Model file for the job. Use its own axes, mm. Face numbers are marked on the shaded views. A direction names the side the tool comes from. Give positions to 0.01 mm unless a question says otherwise; leave off trailing zeros. Loops run counter-clockwise (first coordinate to the right, second up) from the corner with the lowest first, then second, coordinate; pieces in that order, holes last. Notation, with made-up numbers: M 26,-34.75 L 35,-34.75 A36 ccw 35,4.25 Z; hole C -20,12.5 d2. An arc over 180 degrees is marked long. Answer in a Markdown table with one row per item.
```python
from build123d import *
from build123d.topology import SkipClean

# Parameters (mm, degrees)
SKETCH_1_R          = 18
SKETCH_1_R_2        = 5
EXTRUDE_1_DEPTH     = 20
SKETCH_2_R          = 10
EXTRUDE_2_DEPTH     = 35
SKETCH_4_R          = 15
SKETCH_4_R_2        = 7.5
CUT_EXTRUDE_3_DEPTH = 28.5


with BuildPart() as part:
    # Эскиз1 → Вытянуть1 (new body)
    with BuildSketch(Plane.XY):
        Circle(SKETCH_1_R)
        Circle(SKETCH_1_R_2, mode=Mode.SUBTRACT)
    extrude(amount=EXTRUDE_1_DEPTH)

    # Эскиз2 → Вытянуть2 (add)
    with SkipClean():  # the faces are left unmerged after this step: merging them gives an invalid solid
        with BuildSketch(Plane(origin=(0, 14, 0), x_dir=(1, 0, 0), z_dir=(0, 1, 0))):
            with Locations(Location((0, -10, 0), (0, 0, 270))):
                Circle(SKETCH_2_R)
        extrude(amount=EXTRUDE_2_DEPTH)

    # Эскиз4 → Вытянуть3 (cut)
    with SkipClean():  # the faces are left unmerged after this step: merging them gives an invalid solid
        with BuildSketch(Plane(origin=(0, 49, 0), x_dir=(1, 0, 0), z_dir=(0, 1, 0))):
            with Locations((0, -10)):
                Circle(SKETCH_4_R)
            with Locations(Location((0, -10, 0), (0, 0, 270))):
                Circle(SKETCH_4_R_2, mode=Mode.SUBTRACT)
        extrude(amount=-CUT_EXTRUDE_3_DEPTH, mode=Mode.SUBTRACT)


solid = part.part
```
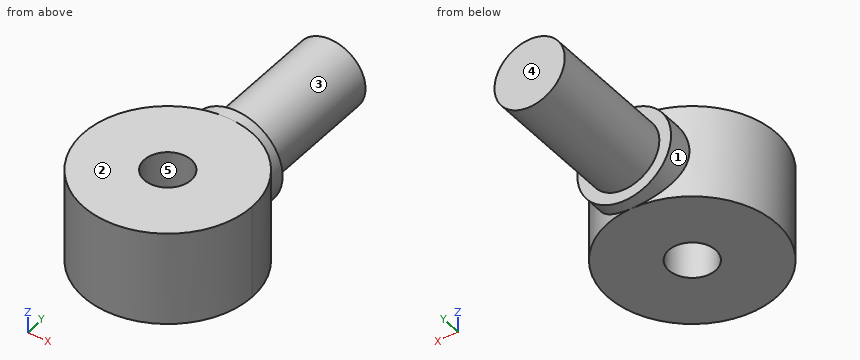
Q1. Saw through at A-A (z = 10). Give the cut face in (x, y), and give its area (3 significant figures).
Reported:
| item | result |
|---|---|
| outline | M -10,14.97 A18 ccw long 10,14.97 L 10,20.5 L 7.5,20.5 L 7.5,49 L -7.5,49 L -7.5,20.5 L -10,20.5 Z; hole C 0,0 d10 |
| area | 1,440 mm² |
Q2. Drop flat-ended pins along their axis: pin 1 (3 mm diameter, centred on y = 31, z = 5.5, fed in from +X); pin 2 (5 mm diameter, centred on y = 19, z = 8, fed in from -X); pin 3 (8 mm diameter, centred on x = 0, y = 0, fed in from +Z); pin 4 (1.5 mm diameter, centred on x = -12.5, z = 5, fed in from +Y). Give the stop position or say it passes through.
Reported:
| item | result |
|---|---|
| pin 1 | x = 6.87 |
| pin 2 | x = -10 |
| pin 3 | through |
| pin 4 | y = 13.64 |
Q3. Saw through at D-D (x = -9). Give the cut face in (y, z), and give its area (3 significant figures).
Reported:
| item | result |
|---|---|
| outline | M -15.59,0 L 15.59,0 L 15.59,5.64 L 20.5,5.64 L 20.5,14.36 L 15.59,14.36 L 15.59,20 L -15.59,20 Z |
| area | 666 mm² |
Q4. Probe probe 1 along Y at (x, z) = (0, 14.5); probe 2 along Y at (x, z) = (-2, 15.75); probe 3 along X at (y, z) = (-1, 11.75). List the from-to ranges inside material, lowest first.
Reported:
| item | result |
|---|---|
| probe 1 | -18 to -5, 5 to 49 |
| probe 2 | -17.89 to -4.58, 4.58 to 49 |
| probe 3 | -17.97 to -4.9, 4.9 to 17.97 |
Q5. Mould opens along Y. For the marked faces 3, 4 and 5 say: released by +Y, released by -Y, zero draft, split by the parting line, or undercut.
Reported:
| item | result |
|---|---|
| face 3 | zero draft |
| face 4 | released by +Y |
| face 5 | undercut |
Q6. Saw through at C-C (y = 19). Give the cut face in (x, z), and give its area (3 significant figures).
Reported:
| item | result |
|---|---|
| outline | C 0,10 d20 |
| area | 314 mm² |
Q7. 3-axis set-ups, long thin cutter, end or side, ignore diameter. For the marked faces 1 and 2: which of +Z, -Z, +X, -X, +Y, -Y reach the whole face in a straight line?
Reported:
| item | result |
|---|---|
| face 1 | +Y |
| face 2 | +Z, +X, -X, +Y, -Y |
Q8. Saw through at B-B (x = -4). Give the cut face in (y, z), and give its area (3 significant figures).
Reported:
| item | result |
|---|---|
| outline | M -17.55,0 L -3,0 L -3,20 L -17.55,20 Z; M 3,0 L 17.55,0 L 17.55,0.83 L 20.5,0.83 L 20.5,3.66 L 49,3.66 L 49,16.34 L 20.5,16.34 L 20.5,19.17 L 17.55,19.17 L 17.55,20 L 3,20 Z |
| area | 998 mm² |
